from build123d import *

# Parameters (mm, degrees)
BOSS_EXTRUDE1_DEPTH = 156.5
SKETCH4_W           = 37.518488727
SKETCH4_H           = 12.5
CUT_EXTRUDE1_DEPTH  = 173.977599706
SKETCH5_W           = 33.314858612
SKETCH5_H           = 28
CUT_EXTRUDE2_DEPTH  = 173.977599706
CUT_EXTRUDE3_DEPTH  = 170.294892232
LPATTERN1_COUNT     = 4
LPATTERN1_PITCH     = 43
CHAMFER3_SIZE       = 7
FILLET1_R           = 8
CHAMFER5_SIZE       = 6
SKETCH7_W           = 42
SKETCH7_H           = 7
CUT_EXTRUDE4_DEPTH  = 1


# Some blends are built 0.0001 mm under size
with BuildPart() as part:
    # Sketch1 → Boss-Extrude1 (new body)
    with BuildSketch(Plane(origin=(0, 0, 0), x_dir=(1, 0, 0), z_dir=(0, 1, 0))):
        Polygon((-9.215122984, 0), (-9.215122984, -10), (-5.215122984, -10), (-5.215122984, 0), (56.784877016, 0), (56.784877016, -10), (60.784877016, -10), (60.784877016, 0), (63.784877016, 0), (59.743425131, 7), (-8.1736711, 7), (-12.215122984, 0), align=None)
    extrude(amount=BOSS_EXTRUDE1_DEPTH)

    # Sketch4 → Cut-Extrude1 (cut, through all)
    with BuildSketch(Plane(origin=(60.784877016, 0, 0), x_dir=(0, 0, -1), z_dir=(1, 0, 0))):
        with Locations((-18.759244364, 150.25)):
            Rectangle(SKETCH4_W, SKETCH4_H)
    extrude(amount=-CUT_EXTRUDE1_DEPTH, mode=Mode.SUBTRACT)

    # Sketch5 → Cut-Extrude2 (cut, through all)
    with BuildSketch(Plane(origin=(60.784877016, 0, 0), x_dir=(0, 0, -1), z_dir=(1, 0, 0))):
        with Locations((-16.657429306, 115)):
            Rectangle(SKETCH5_W, SKETCH5_H)
    cut_extrude2 = extrude(amount=-CUT_EXTRUDE2_DEPTH, mode=Mode.SUBTRACT)

    # Sketch6 → Cut-Extrude3 (cut, symmetric)
    with BuildSketch(Plane(origin=(0, 0, 0), x_dir=(0, 0, -1), z_dir=(1, 0, 0))):
        Polygon((-7.3, 137.827905619), (-6.15, 138.491858429), (-10, 138.491858429), (-10, 134.508141571), (-6.15, 134.508141571), (-7.3, 135.172094381), align=None)
        Polygon((-5, 133.844188762), (-2.7, 135.172094381), (-2.7, 137.827905619), (-5, 139.155811238), (-7.3, 137.827905619), (-7.3, 135.172094381), align=None)
    cut_extrude3 = extrude(amount=CUT_EXTRUDE3_DEPTH, both=True, mode=Mode.SUBTRACT)

    # LPattern1: Cut-Extrude2, Cut-Extrude3 ×4
    with Locations(*[(0, -i * LPATTERN1_PITCH, 0) for i in range(1, LPATTERN1_COUNT)]):
        add(cut_extrude2, mode=Mode.SUBTRACT)
        add(cut_extrude3, mode=Mode.SUBTRACT)

    # Chamfer3
    chamfer3_edges = [part.edges().sort_by_distance(p)[0] for p in [
        (25.784877016, 156.5, -7),
    ]]
    chamfer(chamfer3_edges, length=CHAMFER3_SIZE - 0.0001)  # a hair under: the kernel refuses the full size

    # Fillet1
    fillet1_edges = [part.edges().sort_by_distance(p)[0] for p in [
        (-8.1736711, 74.75005, -7),
        (59.743425131, 74.75005, -7),
    ]]
    fillet(fillet1_edges, radius=FILLET1_R)

    # Chamfer5
    # the kernel refuses this chamfer: 6 mm, written as the material it takes off along each edge
    with BuildSketch(Plane(origin=(76.214974943, 43, 10), x_dir=(0, -0.027495876610586778, -0.9996219169112968), z_dir=(-1, 0, 0)), Plane(origin=(41.354779088, 144, 10), x_dir=(0, 0.027495876610586778, -0.9996219169112968), z_dir=(1, 0, 0)), Plane(origin=(76.214974943, 129, 10), x_dir=(0, -0.027495876610586778, -0.9996219169112968), z_dir=(-1, 0, 0)), Plane(origin=(-24.645220912, 144, 10), x_dir=(0, 0.027495876610586775, -0.9996219169112968), z_dir=(1, 0, 0)), Plane(origin=(10.214974943, 129, 10), x_dir=(0, -0.027495876610586778, -0.9996219169112968), z_dir=(-1, 0, 0)), Plane(origin=(-24.645220912, 101, 10), x_dir=(0, 0.027495876610586775, -0.9996219169112968), z_dir=(1, 0, 0)), Plane(origin=(10.214974943, 86, 10), x_dir=(0, -0.027495876610586778, -0.9996219169112968), z_dir=(-1, 0, 0)), Plane(origin=(41.354779088, 101, 10), x_dir=(0, 0.027495876610586778, -0.9996219169112968), z_dir=(1, 0, 0)), Plane(origin=(76.214974943, 86, 10), x_dir=(0, -0.027495876610586778, -0.9996219169112968), z_dir=(-1, 0, 0)), Plane(origin=(41.354779088, 58, 10), x_dir=(0, 0.027495876610586778, -0.9996219169112968), z_dir=(1, 0, 0)), Plane(origin=(41.354779088, 15, 10), x_dir=(0, 0.02749587661058649, -0.9996219169112968), z_dir=(1, 0, 0)), Plane(origin=(-24.645220912, 15, 10), x_dir=(0, 0.027495876610586487, -0.9996219169112968), z_dir=(1, 0, 0)), Plane(origin=(-24.645220912, 58, 10), x_dir=(0, 0.027495876610586775, -0.9996219169112968), z_dir=(1, 0, 0)), Plane(origin=(10.214974943, 43, 10), x_dir=(0, -0.027495876610586778, -0.9996219169112968), z_dir=(-1, 0, 0))) as chamfer5_piece_1:
        Polygon((CHAMFER5_SIZE * 0.999621916911, -CHAMFER5_SIZE * 0.0274958766106), (-CHAMFER5_SIZE * 0.0274958766106, -CHAMFER5_SIZE * 0.999621916911), (0, 0), align=None)
    extrude(amount=34.860195856, mode=Mode.SUBTRACT)
    with BuildSketch(Plane(origin=(41.354779088, 0, 10), x_dir=(0, -0.027495876610586372, -0.9996219169112968), z_dir=(1, 0, 0)), Plane(origin=(-24.645220912, 0, 10), x_dir=(0, -0.027495876610586372, -0.9996219169112968), z_dir=(1, 0, 0))) as chamfer5_piece_2:
        Polygon((CHAMFER5_SIZE * 0.999621916911, CHAMFER5_SIZE * 0.0274958766106), (-CHAMFER5_SIZE * 0.0274958766106, CHAMFER5_SIZE * 0.999621916911), (0, 0), align=None)
    extrude(amount=34.860195856, mode=Mode.SUBTRACT)

    # Sketch7 → Cut-Extrude4 (cut)
    with BuildSketch(Plane(origin=(0, 0, -7), x_dir=(-1, 0, 0), z_dir=(0, 0, -1))):
        with Locations((-25.784877016, 94.957259422)):
            Rectangle(SKETCH7_W, SKETCH7_H)
        Polygon((-25.784877016, 79.332903769), (-4.784877016, 91.457259422), (-18.784877016, 91.457259422), (-25.784877016, 87.415807537), (-32.784877016, 91.457259422), (-46.784877016, 91.457259422), (-32.784877016, 83.374355653), align=None)
        Polygon((-32.784877016, 75.291451884), (-25.784877016, 79.332903769), (-32.784877016, 83.374355653), (-46.784877016, 75.291451884), (-32.784877016, 67.208548116), (-25.784877016, 71.25), align=None)
        with BuildLine():
            Line((-18.784877016, 75.291451884), (-25.784877016, 71.25))
            Line((-25.784877016, 71.25), (-32.784877016, 67.208548116))
            Line((-32.784877016, 67.208548116), (-46.784877016, 59.125644347))
            Line((-46.784877016, 59.125644347), (-46.784877016, 51.042740578))
            Line((-46.784877016, 51.042740578), (-25.784877016, 63.167096231))
            Line((-25.784877016, 63.167096231), (-25.784877016, 61.542740578))
            ThreePointArc((-25.784877016, 61.542740578), (-15.284877016, 51.042740578), (-4.784877016, 61.542740578))
            Line((-4.784877016, 61.542740578), (-4.784877016, 83.374355653))
            Line((-4.784877016, 83.374355653), (-11.784877016, 79.332903769))
            Line((-11.784877016, 79.332903769), (-11.784877016, 61.542740578))
            ThreePointArc((-11.784877016, 61.542740578), (-15.284877016, 58.042740578), (-18.784877016, 61.542740578))
            Line((-18.784877016, 61.542740578), (-18.784877016, 75.291451884))
        make_face()
    extrude(amount=-CUT_EXTRUDE4_DEPTH, mode=Mode.SUBTRACT)


solid = part.part
Can you work these out from the model? Positions are in its coordinate system, mm. A direction names the side the tool comes from. Give positions to 0.01 mm unless a question says otherwise; leave off trailing zeros. Order: outer loops, then holes, each group sorted by start corner. A loop starts at its lowest first (then second) coordinate and runs counter-clockwise, first axis right, second up. Notation, with made-up numbers: M -34,-32 L -20,-32 A21 cw -20,1 Z; hole C 30.25,-17.5 d6. An arc over 180 degrees is marked long. One line per question, with ' | ' between items.
Item 1: Suppose I cut it at C-C, the plane z = 8. Give the number of separate pieces and of enclosed holes in the cut face, then the cut area to 3 significant figures.
Answer block:
separate pieces: 16 | enclosed holes: 0 | area: 96.5 mm2
Item 2: Suppose I cut it at A-A, the plane y = 45. Write out the boundary of the cut face in (x, z), then the cut area to 3 significant figures.
Answer block:
outline: M -12.22,0 L -10.48,-3 A8 ccw -3.55,-7 L 55.12,-7 A8 ccw 62.05,-3 L 63.78,0 L 60.78,0 L 60.78,6 L 56.78,6 L 56.78,0 L -5.22,0 L -5.22,6 L -9.22,6 L -9.22,0 Z | area: 545 mm2
Item 3: I'm going to push flat-ended pins straight in: pin 1 Ø3 at (x, z) = (17, -5) entering from +Y; pin 2 Ø1.1 at (y, z) = (95.5, -6.5) entering from +X; pin 3 Ø6 at (y, z) = (37.5, -1.5) entering from +X. Where does each tip first touch, or does it pass through?
Answer block:
pin 1: stops at y = 153 | pin 2: stops at x = 59.09 | pin 3: stops at x = 63.78
Item 4: For faces 5 (the face through (-7, 50, 2.7)), 6 (the face through (-7, 144, 2)), 7 (the face through (25, 77, 0)), which set-ups out of +Z, -Z, +X, -X, +Y, -Y let a thin tool reach every point of the face, with its end or its side?
Answer block:
face 5: +Z, +X, -X | face 6: +Z, +X, -X, +Y | face 7: +Z
Item 5: We'd pull the mould along X, two halves only. Please class faces 1 (the face through (59, 136, 2.7)), 2 (the face through (29.236, 73.242, -6.507)), 3 (the face through (39.69, 63.22, -6.51)), 4 (the face through (-9.215, 50, 2)): released by +X, released by -X, zero draft, split by the parting line, or undercut.
Answer block:
face 1: zero draft | face 2: undercut | face 3: undercut | face 4: released by -X
Item 6: Please list where these lines run through material, in increasing order: L1, parallel to X at y = 13, z = 0.5; L2, parallel to Z at x = 13, y = 75; L3, parallel to Z at x = 5, y = 93.5.
Answer block:
L1: x = -9.22 to -5.22, 56.78 to 60.78 | L2: z = -7 to 0 | L3: z = -6 to 0
